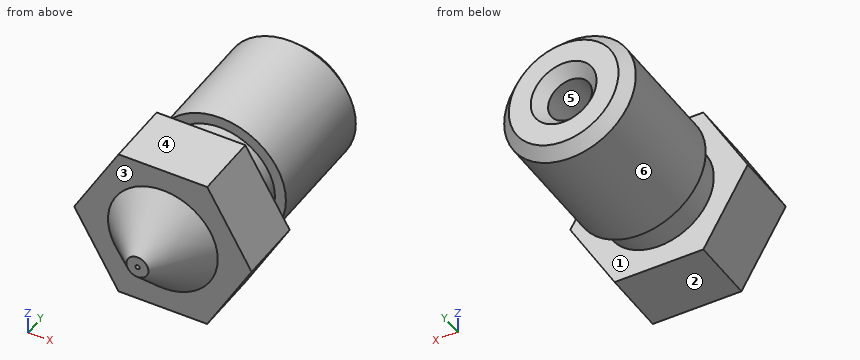
from build123d import *

# Parameters (mm, degrees)
BOSS_EXTRUDE1_DEPTH = 3
CHAMFER1_SIZE       = 0.5


with BuildPart() as part:
    # Sketch1 → Boss-Extrude1 (new body)
    with BuildSketch(Plane.XZ):
        Polygon((-2.020725942, 3.5), (-4.041451884, 0), (-2.020725942, -3.5), (2.020725942, -3.5), (4.041451884, 0), (2.020725942, 3.5), align=None)
    extrude(amount=-BOSS_EXTRUDE1_DEPTH)

    # Sketch2 → Revolve1 (revolve)
    with BuildSketch(Plane(origin=(0, 0, 0), x_dir=(-1, 0, 0), z_dir=(0, 0, -1))):
        Polygon((-2.5, 3), (0, 3), (0, 10.5), (-3, 10.5), (-3, 4.5), (-2.5, 4.5), align=None)
    revolve(axis=Axis((0, 3, 0), (0, 1, 0)))

    # Sketch3 → Revolve2 (revolve)
    with BuildSketch(Plane.XY):
        Polygon((2.5, 0), (0, 0), (0, -2), (0.5, -2), align=None)
    revolve(axis=Axis((0, 0, 0), (0, -1, 0)))

    # Sketch4 → Cut-Revolve1 (revolve, cut)
    with BuildSketch(Plane(origin=(0, 0, 0), x_dir=(-1, 0, 0), z_dir=(0, 0, -1))):
        Polygon((-0.1, -2), (0, -2), (0, 10.5), (-1, 10.5), (-1, 0), (-0.75, -0.227272727), (-0.75, -0.7), (-0.1, -1.2), align=None)
    revolve(axis=Axis((0, -2, 0), (0, 1, 0)), mode=Mode.SUBTRACT)

    # Chamfer1
    chamfer1_edges = [part.edges().sort_by_distance(p)[0] for p in [
        (-3, 10.5, 0),
        (-1, 10.5, 0),
    ]]
    chamfer(chamfer1_edges, length=CHAMFER1_SIZE)


solid = part.part
Model file for the job. Use its own axes, mm. Face numbers are marked on the shaded views. A direction names the side the tool comes from. Coordinates: 2 decimals unless noted, no trailing zeros. Order: outer loops, then holes, each group sorted by start corner. A loop starts at its lowest first (then second) coordinate and runs counter-clockwise, first axis right, second up. Notation, with made-up numbers: M -26,40 L 19,40 A16 ccw 19,45 Z; hole C 18,53.5 d11. An arc over 180 degrees is marked long. Return JSON: item names as keys, results as strings.
1. Tool access for the marked faces 1, 2 and 3: list every direction of +Z, -Z, +X, -X, +Y, -Y with a clear straight run to the whole face (end or side of a thin tool).
Ans:
{"face 1": "none", "face 2": "-Z, +X, -X, +Y, -Y", "face 3": "-Y"}
2. Flat gauge pins, fed straight in: pin 1 (2 mm diameter, centred on y = 2, z = 0.5, fed in from +X); pin 2 (3 mm diameter, centred on x = 0.5, y = 7.5, fed in from -Z); pin 3 (1.8 mm diameter, centred on x = -1, z = -1.5, fed in from -Y); pin 4 (3.5 mm diameter, centred on x = -1, z = -0.5, fed in from -Y). Where does each tip first touch, or does it go through?
Ans:
{"pin 1": "x = 4.04", "pin 2": "z = -3", "pin 3": "y = -1.6", "pin 4": "y = -2"}
3. Saw through at A-A (y = 8). Give the cut face in (x, z).
Ans:
{"outline": "C 0,0 d6; hole C 0,0 d2"}
4. Drill centre lines: probe 1 along Z at (x, y) = (0, -1.75); probe 2 along Z at (x, y) = (0, 9); probe 3 along Y at (x, z) = (3.25, 0.5). Where is each one in solid material? Low to high.
Ans:
{"probe 1": "-0.75 to -0.1, 0.1 to 0.75", "probe 2": "-3 to -1, 1 to 3", "probe 3": "0 to 3"}
5. Pull direction X, two halves, no side cores. Call the marked faces 4, 5 and 6: +X half, -X half, draft (parallel to the pull), parting line (faces both ways), or undercut.
Ans:
{"face 4": "draft", "face 5": "undercut", "face 6": "parting line"}
